from build123d import *

# Parameters (mm, degrees)
SKETCH_1_W          = 30
SKETCH_1_H          = 20
EXTRUDE_1_DEPTH     = 30
SKETCH_2_W          = 6
SKETCH_2_H          = 5
CUT_EXTRUDE_1_DEPTH = 30
CUT_EXTRUDE_2_DEPTH = 30
SKETCH_4_W          = 5
SKETCH_4_H          = 4
CUT_EXTRUDE_3_DEPTH = 4
SKETCH_6_W          = 16
SKETCH_6_H          = 5
CUT_EXTRUDE_4_DEPTH = 10


with BuildPart() as part:
    # 草圖1 → 填料-伸長1 (new body)
    with BuildSketch(Plane.XY):
        Rectangle(SKETCH_1_W, SKETCH_1_H)
    extrude(amount=EXTRUDE_1_DEPTH)

    # 草圖2 → 除料-伸長1 (cut)
    with BuildSketch(Plane.XY.offset(30)):
        with Locations((-2, -7.5)):
            Rectangle(SKETCH_2_W, SKETCH_2_H)
    extrude(amount=-CUT_EXTRUDE_1_DEPTH, mode=Mode.SUBTRACT)

    # 草圖3 → 除料-伸長2 (cut)
    with BuildSketch(Plane.XY.offset(30)):
        Polygon((-10, 10), (-10, -5.551195207), (15, 10), align=None)
    extrude(amount=-CUT_EXTRUDE_2_DEPTH, mode=Mode.SUBTRACT)

    # 草圖4 → 除料-伸長3 (cut)
    with BuildSketch(Plane(origin=(0, 10, 0), x_dir=(1, 0, 0), z_dir=(0, 1, 0))):
        with Locations((-12.5, -22)):
            Rectangle(SKETCH_4_W, SKETCH_4_H)
    extrude(amount=-CUT_EXTRUDE_3_DEPTH, mode=Mode.SUBTRACT)

    # 草圖6 → 除料-伸長4 (cut)
    with BuildSketch(Plane(origin=(0, 10, 0), x_dir=(1, 0, 0), z_dir=(0, 1, 0))):
        with Locations((7, -6.5)):
            Rectangle(SKETCH_6_W, SKETCH_6_H)
    extrude(amount=-CUT_EXTRUDE_4_DEPTH, mode=Mode.SUBTRACT)


solid = part.part
Input: part model. Units: mm. Frame: model coordinates. A direction names the side the tool comes from. Round coordinates to 2 decimals unless told otherwise and drop trailing zeros. Write each loop counter-clockwise with the first axis right and the second up, starting at its lowest first coordinate (ties: lowest second). Pieces come first, ordered by that corner, then holes.
1) Cut plane B-B (y = -1). Return the cut outline in (x, z), then the cut area to 3 significant figures.
2) Draft query along X for faces 6 (the flat face through (-10, 2, 15)), 7 (the flat face through (-13, 10, 27)), 8 (the flat face through (15, 0, 15)). Return one class per face: pulls with the +X half, pulls with the -X half, needs draft (parallel to the pull), parting line crosses it, or undercut.
3) Cut plane C-C (x = 4). Return the cut outline in (y, z).
4) Cut plane A-A (z = 18). Return the cut outline in (x, y).
5) Cut plane D-D (x = 11.5). Return the cut outline in (y, z).
6) Contact query for flat-ended pins moving along their axis: P1, Ø1, axis at x = -6, z = 15, coming from the +Y side; P2, Ø1.5, axis at x = 9, z = 6.5, coming from the +Y side; P3, Ø1, axis at x = -5.5, z = 13, coming from the +Y side. Output: stop coordinate, or through.
7) Reachability of faces 1 (the flat face through (10, 3, 9)), 2 (the flat face through (-13, 8, 24)), 3 (the flat face through (-5, -8, 15)), 4 (the flat face through (-10, -10, 15)), 5 (the flat face through (2.3, 2.1, 15.2)) from +Z, -Z, +X, -X, +Y, -Y: full face, straight path, thin tool, end or side. Return the list, or none.
8) Ray query, L1, parallel to Z at x = 7.5, y = 0.5; L2, parallel to X at y = -7.25, z = 16; L3, parallel to X at y = 8.75, z = 3.25. Return the intervals inside material, ascending.
Geometry says:
1. outline: (-15, 0) - (-10, 0) - (-10, 30) - (-15, 30) - close; (-2.68, 0) - (15, 0) - (15, 30) - (-2.68, 30) - close
1. area: 681 mm2
2. face 6: undercut
2. face 7: needs draft
2. face 8: pulls with the +X half
3. outline: (-10, 0) - (3.16, 0) - (3.16, 4) - (0, 4) - (0, 9) - (3.16, 9) - (3.16, 30) - (-10, 30) - close
4. outline: (-15, -10) - (-5, -10) - (-5, -5) - (1, -5) - (1, -10) - (15, -10) - (15, 10) - (-10, -5.55) - (-10, 10) - (-15, 10) - close
5. outline: (-10, 0) - (7.82, 0) - (7.82, 4) - (0, 4) - (0, 9) - (7.82, 9) - (7.82, 30) - (-10, 30) - close
6. P1: stops at y = -2.75
6. P2: stops at y = 0
6. P3: stops at y = -2.44
7. face 1: +X, +Y
7. face 2: -X, +Y
7. face 3: +Z, -Z, -Y
7. face 4: +Z, -Z, +X, -X, -Y
7. face 5: +Z, -Z, +Y
8. L1: z = 0 to 4, 9 to 30
8. L2: x = -15 to -5, 1 to 15
8. L3: x = -15 to -10, 12.99 to 15
